```python
from build123d import *

# Parameters (mm, degrees)
SKETCH003_W      = 15
SKETCH003_H      = 3
EXTRUDE003_DEPTH = 18
SKETCH002_W      = 119.97
SKETCH002_H      = 73.25
SKETCH002_R      = 1.45
SKETCH002_W_2    = 14
SKETCH002_H_2    = 14
SKETCH002_W_3    = 23.344
SKETCH002_H_3    = 11.824
EXTRUDE002_DEPTH = 3
FILLET001_R      = 5


with BuildPart() as extrude003:
    # Sketch003 (on Face4 of Extrude002) → Extrude003 (new body)
    with BuildSketch(Plane(origin=(0, 63.25, 0), x_dir=(-1, 0, 0), z_dir=(0, 1, 0))):
        with Locations((-45.204, 23.5)):
            Rectangle(SKETCH003_W, SKETCH003_H)
    extrude(amount=-EXTRUDE003_DEPTH)


with BuildPart() as fillet001:
    # Sketch002 (on Face14 of Extrude001) → Extrude002 (new body)
    with BuildSketch(Plane.XY.offset(22)):
        with Locations((49.985, 26.625)):
            Rectangle(SKETCH002_W, SKETCH002_H)
        with Locations((104.97, -5)):
            Circle(SKETCH002_R, mode=Mode.SUBTRACT)
        with Locations((104.97, 58.25)):
            Circle(SKETCH002_R, mode=Mode.SUBTRACT)
        with Locations((-5, 58.25)):
            Circle(SKETCH002_R, mode=Mode.SUBTRACT)
        with Locations((-5, -5)):
            Circle(SKETCH002_R, mode=Mode.SUBTRACT)
        with Locations((87.902, 10.673)):
            Rectangle(SKETCH002_W_2, SKETCH002_H_2, mode=Mode.SUBTRACT)
        with Locations((68.896, 10.673)):
            Rectangle(SKETCH002_W_2, SKETCH002_H_2, mode=Mode.SUBTRACT)
        with Locations((49.89, 10.673)):
            Rectangle(SKETCH002_W_2, SKETCH002_H_2, mode=Mode.SUBTRACT)
        with Locations((30.884, 10.673)):
            Rectangle(SKETCH002_W_2, SKETCH002_H_2, mode=Mode.SUBTRACT)
        with Locations((11.878, 10.673)):
            Rectangle(SKETCH002_W_2, SKETCH002_H_2, mode=Mode.SUBTRACT)
        with Locations((78.22, 35.956)):
            Rectangle(SKETCH002_W_2, SKETCH002_H_2, mode=Mode.SUBTRACT)
        with Locations((16.038, 39.718)):
            Rectangle(SKETCH002_W_3, SKETCH002_H_3, mode=Mode.SUBTRACT)
    extrude(amount=EXTRUDE002_DEPTH)

    # Cut: cut Extrude003
    add(extrude003.part, mode=Mode.SUBTRACT)

    # Fillet001
    fillet001_edges = [fillet001.edges().sort_by_distance(p)[0] for p in [
        (-10, 63.25, 23.5),
        (-10, -10, 23.5),
        (109.97, -10, 23.5),
        (109.97, 63.25, 23.5),
    ]]
    fillet(fillet001_edges, radius=FILLET001_R)


solid = fillet001.part
```
Check sheet for the modelled part. Datum: model origin and axes. Units: mm. A direction names the side the tool comes from. Coordinates: 2 decimals unless noted, no trailing zeros. Order: outer loops, then holes, each group sorted by start corner. A loop starts at its lowest first (then second) coordinate and runs counter-clockwise, first axis right, second up. Notation, with made-up numbers: M 86.5,50 L 135.5,50 A18 ccw 135.5,81 Z; hole C 21.5,45.5 d6. An arc over 180 degrees is marked long. One line per question, with ' | ' between items. Start each with the question number.
Item 1: Sectioned sample at D-D on x = 22.5. Record the cut outline in (y, z), and give its area (3 significant figures).
Item 2: Sectioned sample at C-C on y = 37.5. Record the cut outline in (x, z).
Item 3: Sectioned sample at A-A on x = 68. Record the cut outline in (y, z).
Item 4: Sectioned sample at B-B on y = 6. Record the cut outline in (x, z), and give its area (3 significant figures).
Item 5: Mould release check, pull along X, two halves, no side actions. Record for faces 4 (the flat face through (94.902, 11, 23)), 5 (the flat face through (109.97, 26, 23)), 6 (the cylindrical face through (-9, -8, 24)): pulls with the +X half, pulls with the -X half, needs draft (parallel to the pull), parting line crosses it, or undercut.
Item 6: Material ranges on line 1 (Y direction, x = 14.5, z = 22.2); line 2 (X direction, y = 15.5, z = 23.8); line 3 (Y direction, x = 104.97, z = 22.7), recorded low to high.
Item 7: Access from +Z, -Z, +X, -X, +Y, -Y to the whole of each face (thin tool, end or side, straight path). Record for faces 1 (the flat face through (45, 45.25, 24)), 2 (the flat face through (37.884, 11, 23)), 3 (the cylindrical face through (-8.57, 61.75, 23.52)).
Answer below:
1) outline: M -10,22 L 33.81,22 L 33.81,25 L -10,25 Z; M 45.63,22 L 63.25,22 L 63.25,25 L 45.63,25 Z | area: 184 mm^2
2) outline: M -10,22 L 4.37,22 L 4.37,25 L -10,25 Z; M 27.71,22 L 71.22,22 L 71.22,25 L 27.71,25 Z; M 85.22,22 L 109.97,22 L 109.97,25 L 85.22,25 Z
3) outline: M -10,22 L 3.67,22 L 3.67,25 L -10,25 Z; M 17.67,22 L 63.25,22 L 63.25,25 L 17.67,25 Z
4) outline: M -10,22 L 4.88,22 L 4.88,25 L -10,25 Z; M 18.88,22 L 23.88,22 L 23.88,25 L 18.88,25 Z; M 37.88,22 L 42.89,22 L 42.89,25 L 37.88,25 Z; M 56.89,22 L 61.9,22 L 61.9,25 L 56.89,25 Z; M 75.9,22 L 80.9,22 L 80.9,25 L 75.9,25 Z; M 94.9,22 L 109.97,22 L 109.97,25 L 94.9,25 Z | area: 150 mm^2
5) face 4: undercut | face 5: pulls with the +X half | face 6: pulls with the -X half
6) line 1: y = -10 to 3.67, 17.67 to 33.81, 45.63 to 63.25 | line 2: x = -10 to 4.88, 18.88 to 23.88, 37.88 to 42.89, 56.89 to 61.9, 75.9 to 80.9, 94.9 to 109.97 | line 3: y = -10 to -6.45, -3.55 to 56.8, 59.7 to 63.25
7) face 1: +Z, -Z, +Y | face 2: +Z, -Z | face 3: +Z, -Z, -X, +Y
